Input: dimensioned drawing with shaded views. Units: mm. Origin: part minimum x, y, z. Give positions to 0.01 mm unless a question says otherwise; leave off trailing zeros. Write each loop counter-clockwise with the first axis right and the second up, starting at its lowest first coordinate (ties: lowest second). Pieces come first, ordered by that corner, then holes.
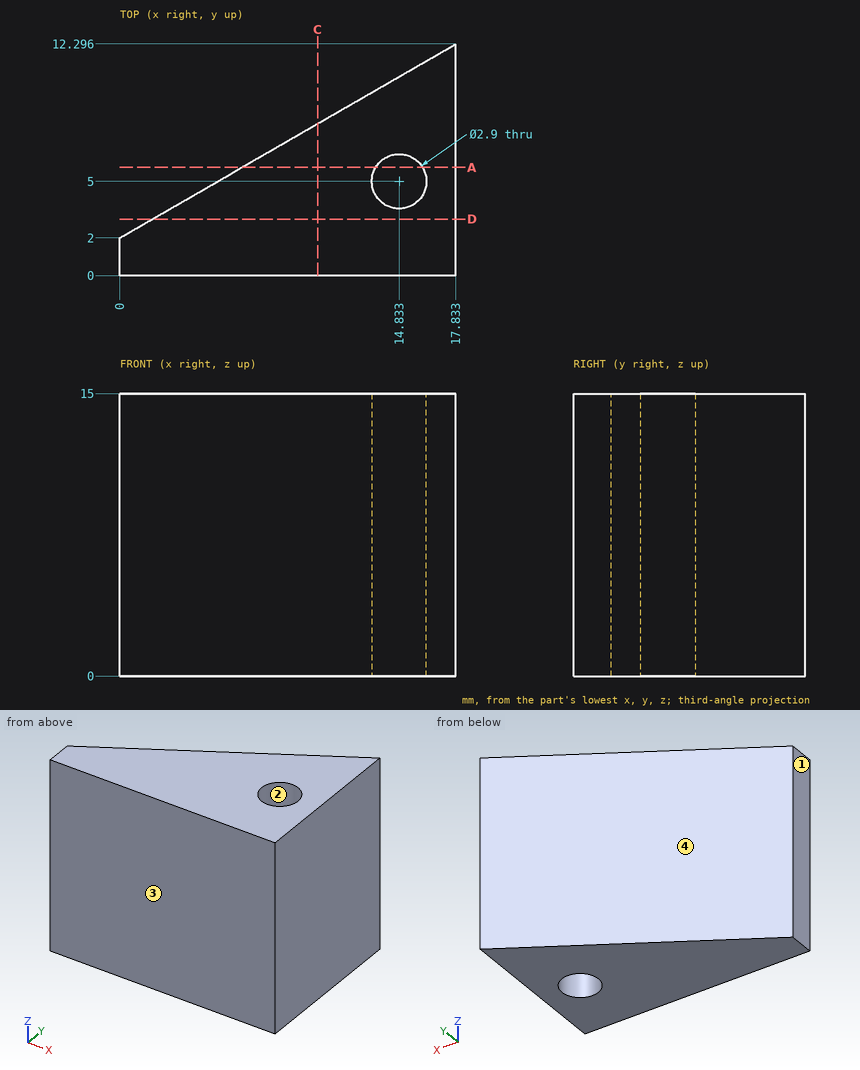
Item 1: Pin query (flat end, axial travel): pin 1 (1 mm diameter, centred on x = 12, z = 6.5, fed in from -Y); pin 2 (6 mm diameter, centred on x = 4.5, y = 10.5, fed in from +Z); pin 3 (3 mm diameter, centred on x = 11.5, z = 9, fed in from +Y) (1 decimal). Return the tip coordinate at first contact, or that it passes through.
Item 2: Ray query, line 1 (X direction, y = 5, z = 3.75) (1 decimal); line 2 (Y direction, x = 13.75, z = 6.25) (1 decimal); line 3 (Y direction, x = 5.5, z = 0.5) (1 decimal). Return the intervals inside material, ascending.
Item 3: Section A-A (y = 5.75). Return loops of the section in (x, z) (1 decimal).
Item 4: Section C-C (x = 10.5). Return loops of the section in (y, z).
Item 5: Mould query, pull axis Y, two halves, no side actions, for the marked faces 1, 2, 3 and 4. Classes: +Y half, -Y half, draft (parallel to the pull), parting line (faces both ways), or undercut.
Item 6: Section D-D (y = 3). Return loops of the section in (x, z).
Solved:
1. pin 1: stops at y = 0
1. pin 2: passes through
1. pin 3: stops at y = 9.5
2. line 1: x = 5.2 to 13.4, 16.3 to 17.8
2. line 2: y = 0 to 4, 6 to 9.9
2. line 3: y = 0 to 5.2
3. outline: (6.5, 0) - (13.6, 0) - (13.6, 15) - (6.5, 15) - close; (16.1, 0) - (17.8, 0) - (17.8, 15) - (16.1, 15) - close
4. outline: (0, 0) - (8.06, 0) - (8.06, 15) - (0, 15) - close
5. face 1: draft
5. face 2: undercut
5. face 3: -Y half
5. face 4: +Y half
6. outline: (1.73, 0) - (17.83, 0) - (17.83, 15) - (1.73, 15) - close
